Geometry check sheet. Reference: the model listing, model coordinates, mm. Face numbers are marked on the shaded views. A direction names the side the tool comes from. Give positions to 0.01 mm unless a question says otherwise; leave off trailing zeros. Loops run counter-clockwise (first coordinate to the right, second up) from the corner with the lowest first, then second, coordinate; pieces in that order, holes last.
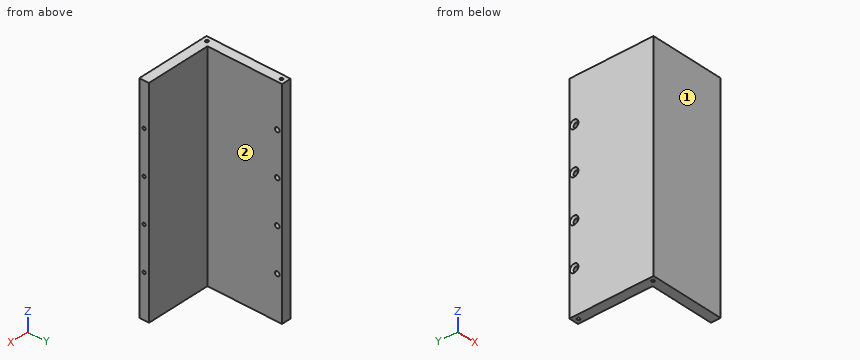
```python
from build123d import *

# Parameters (mm, degrees)
BOSS_EXTRUDE_EQUERRE_DEPTH                     = 113
FRAISAGE_POUR_VIS_T_TE_FRAIS_E_M20_D           = 2.4
FRAISAGE_POUR_VIS_T_TE_FRAIS_E_M20_DEPTH       = 5
FRAISAGE_POUR_VIS_T_TE_FRAIS_E_M20_CSINK_D     = 4.4
FRAISAGE_POUR_VIS_T_TE_FRAIS_E_M20_CSINK_ANGLE = 90
FRAISAGE_POUR_VIS_T_TE_FRAIS_E_M20_TIP         = 0.721032743
TROU_TARAUD_M2X0_43_D                          = 1.6
TROU_TARAUD_M2X0_43_DEPTH                      = 8
TROU_TARAUD_M2X0_43_TIP                        = 0.480688495
TROU_TARAUD_M2X0_44_AT_2_COUNT                 = 2
TROU_TARAUD_M2X0_44_AT_2_PITCH                 = 39


with BuildPart() as part:
    # Esquisse1 → Boss_Extrude_Equerre (new body)
    with BuildSketch(Plane(origin=(0, 0, 0), x_dir=(0, 1, 0), z_dir=(0, 0, 1))):
        Polygon((0, 0), (39, 0), (39, 5), (-5, 5), (-5, 0), (-5, -34), (0, -34), align=None)
    extrude(amount=BOSS_EXTRUDE_EQUERRE_DEPTH)

    # Fraisage pour vis à tête fraisée M20
    with Locations(Plane.ZY.offset(5)):
        with Locations((67.8, 36.5), (90.4, 36.5), (45.2, 36.5), (22.6, 36.5)):
            CounterSinkHole(FRAISAGE_POUR_VIS_T_TE_FRAIS_E_M20_D / 2, FRAISAGE_POUR_VIS_T_TE_FRAIS_E_M20_CSINK_D / 2, depth=FRAISAGE_POUR_VIS_T_TE_FRAIS_E_M20_DEPTH, counter_sink_angle=FRAISAGE_POUR_VIS_T_TE_FRAIS_E_M20_CSINK_ANGLE)
            with Locations((0, 0, -(FRAISAGE_POUR_VIS_T_TE_FRAIS_E_M20_DEPTH + FRAISAGE_POUR_VIS_T_TE_FRAIS_E_M20_TIP / 2))):  # 118° drill point
                Cone(0, FRAISAGE_POUR_VIS_T_TE_FRAIS_E_M20_D / 2, FRAISAGE_POUR_VIS_T_TE_FRAIS_E_M20_TIP, mode=Mode.SUBTRACT)

    # Trou taraudé M2x0.43
    with Locations(Plane.YZ.offset(34)):
        with Locations((-2.5, 67.8), (-2.5, 90.4), (-2.5, 45.2), (-2.5, 22.6)):
            Hole(TROU_TARAUD_M2X0_43_D / 2, depth=TROU_TARAUD_M2X0_43_DEPTH)
            with Locations((0, 0, -(TROU_TARAUD_M2X0_43_DEPTH + TROU_TARAUD_M2X0_43_TIP / 2))):  # 118° drill point
                Cone(0, TROU_TARAUD_M2X0_43_D / 2, TROU_TARAUD_M2X0_43_TIP, mode=Mode.SUBTRACT)

    # Esquisse11 → Trou taraudé M2x0.44 (revolve, cut)
    with BuildSketch(Plane(origin=(-2.5, 36.5, 113), x_dir=(0, -1, 0), z_dir=(1, 0, 0))):
        Polygon((0, 0), (0, 8.480688495), (0.8, 8), (0.8, 0), align=None)
    trou_taraud_m2x0_44 = revolve(axis=Axis((-2.5, 36.5, 119.35), (0, 0, -1)), mode=Mode.SUBTRACT)

    # Trou taraudé M2x0.44 at 2: Trou taraudé M2x0.44 ×2
    with Locations(*[(0, -i * TROU_TARAUD_M2X0_44_AT_2_PITCH, 0) for i in range(1, TROU_TARAUD_M2X0_44_AT_2_COUNT)]):
        add(trou_taraud_m2x0_44, mode=Mode.SUBTRACT)

    # Symétrie1: Trou taraudé M2x0.44 across plane
    add(trou_taraud_m2x0_44.mirror(Plane.XY.offset(56.5)), mode=Mode.SUBTRACT)

    # Symétrie1 copy 1 sketch → Symétrie1 copy 1 (revolve, cut)
    with BuildSketch(Plane(origin=(-2.5, -2.5, 0), x_dir=(0, -1, 0), z_dir=(1, 0, 0))):
        Polygon((0, 0), (0, -8.480688495), (0.8, -8), (0.8, 0), align=None)
    revolve(axis=Axis((-2.5, -2.5, -6.35), (0, 0, -1)), mode=Mode.SUBTRACT)


solid = part.part
```
1) Sectioned sample at B-B on y = 30. Enter the section's corners in (x, z), plus the area to 3 significant figures.
2) Tool access check on the marked faces 1 and 2. Record the directions out of +Z, -Z, +X, -X, +Y, -Y that give a thin tool (end or side, any length) a straight path to the whole face; none if there is none.
3) Sectioned sample at A-A on z = 19. Enter the section's corners in (x, y), plus the area to 3 significant figures.
4) Scan lines: line 1 along X through (y, z) = (36.5, 106.5); line 2 along Y through (x, z) = (-2, 2). Record each from-to range of solid material in increasing order.
5) Depth check by flat-ended pin: P1, Ø2, axis at y = 22, z = 82.5, coming from the +X side; P2, Ø1.4, axis at y = 36.5, z = 67.8, coming from the +X side; P3, Ø1.5, axis at x = 25, z = 45.5, coming from the +Y side; P4, Ø3, axis at y = 36.5, z = 22.6, coming from the -X side. Enter the tip coordinate at first touch or a pass-through.
Determined:
1. outline: (-5, 0) - (0, 0) - (0, 113) - (-5, 113) - close
1. area: 565 mm2
2. face 1: +Z, -Z, +X, -X, -Y
2. face 2: +Z, -Z, +X, +Y
3. outline: (-5, -5) - (34, -5) - (34, 0) - (0, 0) - (0, 39) - (-5, 39) - close
3. area: 390 mm2
4. line 1: x = -5 to -3.3, -1.7 to 0
4. line 2: y = -5 to -3.12, -1.88 to 35.88, 37.12 to 39
5. P1: stops at x = 0
5. P2: passes through
5. P3: stops at y = 0
5. P4: stops at x = -4.3
